from build123d import *

# Parameters (mm, degrees)
BOSS_EXTRUDE1_DEPTH     = 9.525
SKETCH3_R               = 0.508
CUT_EXTRUDE2_DEPTH      = 6.35
FILLET1_R               = 1.5875
ESQUISSE1_W             = 6.35
ESQUISSE1_H             = 6.35
BOSS_EXTRU_1_DEPTH      = 6.35
ESQUISSE2_W             = 7
ESQUISSE2_H             = 5
BOSS_EXTRU_2_DEPTH      = 15
ESQUISSE3_R             = 1.1
ENL_V_MAT_EXTRU_1_DEPTH = 58.756287679
CONG_1_R                = 2.54


with BuildPart() as part:
    # Sketch1 → Boss-Extrude1 (new body)
    with BuildSketch(Plane(origin=(0, 0, 0), x_dir=(0, 0, -1), z_dir=(1, 0, 0))):
        Polygon((0, 0), (12.7847852, 0), (12.7847852, 13.390245), (36.0778552, 13.390245), (36.0778552, 0), (48.8626404, 0), (48.8626404, 4.7625), (42.4278552, 4.7625), (42.4278552, 19.740245), (41.4309052, 19.740245), (6.3509652, 19.740245), (6.3509652, 4.7625), (0, 4.7625), align=None)
    extrude(amount=BOSS_EXTRUDE1_DEPTH)

    # Sketch3 → Cut-Extrude2 (cut)
    with BuildSketch(Plane.ZY):
        with Locations((-38.3232152, 6.68528)):
            Circle(SKETCH3_R)
        with Locations((-10.5229152, 6.6951225)):
            Circle(SKETCH3_R)
    extrude(amount=-CUT_EXTRUDE2_DEPTH, mode=Mode.SUBTRACT)

    # Fillet1
    fillet1_edges = [part.edges().sort_by_distance(p)[0] for p in [
        (4.7625, 4.7625, 0),
        (4.7625, 4.7625, -6.3509652),
        (4.7625, 19.740245, -6.3509652),
        (4.7625, 19.740245, -42.4278552),
        (4.7625, 4.7625, -42.4278552),
        (4.7625, 4.7625, -48.8626404),
    ]]
    fillet(fillet1_edges, radius=FILLET1_R)

    # Esquisse1 → Boss.-Extru.1 (add)
    with BuildSketch(Plane.XZ):
        with Locations((4.7625, -42.4702478)):
            Rectangle(ESQUISSE1_W, ESQUISSE1_H)
        with Locations((4.7625, -6.3923926)):
            Rectangle(ESQUISSE1_W, ESQUISSE1_H)
    extrude(amount=BOSS_EXTRU_1_DEPTH)

    # Esquisse2 → Boss.-Extru.2 (add)
    with BuildSketch(Plane(origin=(-5.859728485, 12.566228289, 0), x_dir=(0, 0, 1), z_dir=(0.4226182617389464, -0.9063077870374674, 0))):
        with Locations((-14.4384652, -12.4751697)):
            Rectangle(ESQUISSE2_W, ESQUISSE2_H)
    extrude(amount=-BOSS_EXTRU_2_DEPTH)

    # Esquisse3 → Enlèv. mat.-Extru.1 (cut, through all)
    with BuildSketch(Plane(origin=(9.040573976, 4.215688879, 0), x_dir=(0, 0, 1), z_dir=(-0.9063077870367755, -0.4226182617404302, 0))):
        with Locations(Location((-14.4384652, 25.865298818, 0), (0, 0, 270))):
            Circle(ESQUISSE3_R)
    extrude(amount=-ENL_V_MAT_EXTRU_1_DEPTH, mode=Mode.SUBTRACT)

    # Congé1
    # the kernel refuses this fillet: 2.54 mm, written as the material it adds along each edge
    with BuildSketch(Plane(origin=(7.318244162, 19.740245, -10.9384652), x_dir=(1, 0, 0), z_dir=(0, 0, -1))) as cong_1_piece_1:
        with BuildLine():
            CenterArc((CONG_1_R * 0.637070260809, -CONG_1_R), CONG_1_R, 90, 65)
            Line((-CONG_1_R * 0.269237526229, -CONG_1_R * 0.577381738261), (0, 0))
            Line((0, 0), (CONG_1_R * 0.637070260809, 0))
        make_face()
    extrude(amount=7)
    with BuildSketch(Plane(origin=(-4.548645433, 19.740245, -10.9384652), x_dir=(0, 0, 1), z_dir=(1, 0, 0))) as cong_1_piece_2_section:
        with BuildLine():
            CenterArc((CONG_1_R, -CONG_1_R), CONG_1_R, 90, 90)
            Line((0, -CONG_1_R), (0, 0))
            Line((0, 0), (CONG_1_R, 0))
        make_face()
    cong_1_piece_2 = extrude(amount=18.216889595, mode=Mode.PRIVATE)
    cong_1_piece_2 = split(cong_1_piece_2, bisect_by=Plane(origin=(5.198744163, 24.285527416, -10.9384652), z_dir=(-0.9063077870374674, -0.4226182617389464, 0)), keep=Keep.TOP, mode=Mode.PRIVATE)
    cong_1_piece_2 = split(cong_1_piece_2, bisect_by=Plane(origin=(0.667205228, 22.172436107, -10.9384652), z_dir=(0.9063077870374674, 0.4226182617389464, 0)), keep=Keep.TOP, mode=Mode.PRIVATE)
    add(cong_1_piece_2)
    with BuildSketch(Plane(origin=(1.801354567, 19.740245, -17.9384652), x_dir=(-1, 0, 0), z_dir=(0, 0, 1))) as cong_1_piece_3:
        with BuildLine():
            CenterArc((3.626366432, -1.766615888), CONG_1_R, 135.931485235, 69.068514765)
            Line((1.324344653, -2.840066273), (0, 0))
            Line((0, 0), (1.801354567, 0))
        make_face()
    extrude(amount=7)
    with BuildSketch(Plane(origin=(13.668244162, 19.740245, -17.9384652), x_dir=(0, 0, -1), z_dir=(-1, 0, 0))) as cong_1_piece_4_section:
        with BuildLine():
            CenterArc((CONG_1_R, -CONG_1_R), CONG_1_R, 90, 90)
            Line((0, -CONG_1_R), (0, 0))
            Line((0, 0), (CONG_1_R, 0))
        make_face()
    cong_1_piece_4 = extrude(amount=18.216889595, mode=Mode.PRIVATE)
    cong_1_piece_4 = split(cong_1_piece_4, bisect_by=Plane(origin=(8.452393501, 17.308053893, -17.9384652), z_dir=(-0.9063077870374674, -0.4226182617389464, 0)), keep=Keep.TOP, mode=Mode.PRIVATE)
    cong_1_piece_4 = split(cong_1_piece_4, bisect_by=Plane(origin=(3.920854566, 15.194962584, -17.9384652), z_dir=(0.9063077870374674, 0.4226182617389464, 0)), keep=Keep.TOP, mode=Mode.PRIVATE)
    add(cong_1_piece_4)
    with BuildSketch(Plane(origin=(7.318244162, 19.740245, -6.893069044), x_dir=(1, 0, 0), z_dir=(0, 0, -1))) as cong_1_piece_5a_section:
        with BuildLine():
            CenterArc((CONG_1_R * 0.637070260809, -CONG_1_R), CONG_1_R, 90, 65)
            Line((-CONG_1_R * 0.269237526229, -CONG_1_R * 0.577381738261), (0, 0))
            Line((0, 0), (CONG_1_R * 0.637070260809, 0))
        make_face()
    cong_1_piece_5a = extrude(amount=11.045396156, mode=Mode.PRIVATE)
    cong_1_piece_5a = split(cong_1_piece_5a, bisect_by=Plane(origin=(7.318244162, 19.740245, -10.9384652), z_dir=(0, 0, 1)), keep=Keep.TOP, mode=Mode.PRIVATE)
    with BuildSketch(Plane(origin=(-4.548645433, 19.740245, -10.9384652), x_dir=(0, 0, 1), z_dir=(1, 0, 0))) as cong_1_piece_5b_section:
        with BuildLine():
            CenterArc((CONG_1_R, -CONG_1_R), CONG_1_R, 90, 90)
            Line((0, -CONG_1_R), (0, 0))
            Line((0, 0), (CONG_1_R, 0))
        make_face()
    cong_1_piece_5b = extrude(amount=18.216889595, mode=Mode.PRIVATE)
    cong_1_piece_5b = split(cong_1_piece_5b, bisect_by=Plane(origin=(9.525, 19.740245, -10.9384652), z_dir=(-1, 0, 0)), keep=Keep.TOP, mode=Mode.PRIVATE)
    cong_1_piece_5b = split(cong_1_piece_5b, bisect_by=Plane(origin=(5.198744163, 24.285527416, -10.9384652), z_dir=(0.9063077870374674, 0.4226182617389464, 0)), keep=Keep.TOP, mode=Mode.PRIVATE)
    cong_1_piece_5 = cong_1_piece_5a & cong_1_piece_5b
    add(cong_1_piece_5)
    with BuildSketch(Plane(origin=(13.668244162, 19.740245, -17.9384652), x_dir=(0, 0, -1), z_dir=(-1, 0, 0))) as cong_1_piece_6a_section:
        with BuildLine():
            CenterArc((CONG_1_R, -CONG_1_R), CONG_1_R, 90, 90)
            Line((0, -CONG_1_R), (0, 0))
            Line((0, 0), (CONG_1_R, 0))
        make_face()
    cong_1_piece_6a = extrude(amount=18.216889595, mode=Mode.PRIVATE)
    cong_1_piece_6a = split(cong_1_piece_6a, bisect_by=Plane(origin=(9.525, 19.740245, -17.9384652), z_dir=(-1, 0, 0)), keep=Keep.TOP, mode=Mode.PRIVATE)
    cong_1_piece_6a = split(cong_1_piece_6a, bisect_by=Plane(origin=(8.452393501, 17.308053893, -17.9384652), z_dir=(0.9063077870374674, 0.4226182617389464, 0)), keep=Keep.TOP, mode=Mode.PRIVATE)
    with BuildSketch(Plane(origin=(7.318244162, 19.740245, -10.9384652), x_dir=(1, 0, 0), z_dir=(0, 0, -1))) as cong_1_piece_6b_section:
        with BuildLine():
            CenterArc((CONG_1_R * 0.637070260809, -CONG_1_R), CONG_1_R, 90, 65)
            Line((-CONG_1_R * 0.269237526229, -CONG_1_R * 0.577381738261), (0, 0))
            Line((0, 0), (CONG_1_R * 0.637070260809, 0))
        make_face()
    cong_1_piece_6b = extrude(amount=11.045396156, mode=Mode.PRIVATE)
    cong_1_piece_6b = split(cong_1_piece_6b, bisect_by=Plane(origin=(7.318244162, 19.740245, -17.9384652), z_dir=(0, 0, -1)), keep=Keep.TOP, mode=Mode.PRIVATE)
    cong_1_piece_6 = cong_1_piece_6a & cong_1_piece_6b
    add(cong_1_piece_6)
    with BuildSketch(Plane(origin=(-4.548645433, 19.740245, -10.9384652), x_dir=(0, 0, 1), z_dir=(1, 0, 0))) as cong_1_piece_7a_section:
        with BuildLine():
            CenterArc((CONG_1_R, -CONG_1_R), CONG_1_R, 90, 90)
            Line((0, -CONG_1_R), (0, 0))
            Line((0, 0), (CONG_1_R, 0))
        make_face()
    cong_1_piece_7a = extrude(amount=18.216889595, mode=Mode.PRIVATE)
    cong_1_piece_7a = split(cong_1_piece_7a, bisect_by=Plane(origin=(0, 19.740245, -10.9384652), z_dir=(1, 0, 0)), keep=Keep.TOP, mode=Mode.PRIVATE)
    cong_1_piece_7a = split(cong_1_piece_7a, bisect_by=Plane(origin=(0.667205228, 22.172436107, -10.9384652), z_dir=(-0.9063077870374674, -0.4226182617389464, 0)), keep=Keep.TOP, mode=Mode.PRIVATE)
    with BuildSketch(Plane(origin=(1.801354567, 19.740245, -17.9384652), x_dir=(-1, 0, 0), z_dir=(0, 0, 1))) as cong_1_piece_7b_section:
        with BuildLine():
            CenterArc((3.626366432, -1.766615888), CONG_1_R, 135.931485235, 69.068514765)
            Line((1.324344653, -2.840066273), (0, 0))
            Line((0, 0), (1.801354567, 0))
        make_face()
    cong_1_piece_7b = extrude(amount=14.834166034, mode=Mode.PRIVATE)
    cong_1_piece_7b = split(cong_1_piece_7b, bisect_by=Plane(origin=(1.801354567, 19.740245, -10.9384652), z_dir=(0, 0, 1)), keep=Keep.TOP, mode=Mode.PRIVATE)
    cong_1_piece_7 = cong_1_piece_7a & cong_1_piece_7b
    add(cong_1_piece_7)
    with BuildSketch(Plane(origin=(13.668244162, 19.740245, -17.9384652), x_dir=(0, 0, -1), z_dir=(-1, 0, 0))) as cong_1_piece_8a_section:
        with BuildLine():
            CenterArc((CONG_1_R, -CONG_1_R), CONG_1_R, 90, 90)
            Line((0, -CONG_1_R), (0, 0))
            Line((0, 0), (CONG_1_R, 0))
        make_face()
    cong_1_piece_8a = extrude(amount=18.216889595, mode=Mode.PRIVATE)
    cong_1_piece_8a = split(cong_1_piece_8a, bisect_by=Plane(origin=(0, 19.740245, -17.9384652), z_dir=(1, 0, 0)), keep=Keep.TOP, mode=Mode.PRIVATE)
    cong_1_piece_8a = split(cong_1_piece_8a, bisect_by=Plane(origin=(3.920854566, 15.194962584, -17.9384652), z_dir=(-0.9063077870374674, -0.4226182617389464, 0)), keep=Keep.TOP, mode=Mode.PRIVATE)
    with BuildSketch(Plane(origin=(1.801354567, 19.740245, -25.772631234), x_dir=(-1, 0, 0), z_dir=(0, 0, 1))) as cong_1_piece_8b_section:
        with BuildLine():
            CenterArc((3.626366432, -1.766615888), CONG_1_R, 135.931485235, 69.068514765)
            Line((1.324344653, -2.840066273), (0, 0))
            Line((0, 0), (1.801354567, 0))
        make_face()
    cong_1_piece_8b = extrude(amount=14.834166034, mode=Mode.PRIVATE)
    cong_1_piece_8b = split(cong_1_piece_8b, bisect_by=Plane(origin=(1.801354567, 19.740245, -17.9384652), z_dir=(0, 0, -1)), keep=Keep.TOP, mode=Mode.PRIVATE)
    cong_1_piece_8 = cong_1_piece_8a & cong_1_piece_8b
    add(cong_1_piece_8)
    # the kernel refuses this fillet: 2.54 mm, written as the material it takes off along each edge
    with BuildSketch(Plane(origin=(7.128164948, 35.173251244, -17.9384652), x_dir=(0, 0, 1), z_dir=(-0.9063077870374675, -0.42261826173894645, 0)), Plane(origin=(-8.913482883, 27.692908011, -10.9384652), x_dir=(0, 0, -1), z_dir=(0.9063077870374675, 0.42261826173894645, 0))) as cong_1_2_piece_1:
        with BuildLine():
            CenterArc((CONG_1_R, -CONG_1_R), CONG_1_R, 90, 90)
            Line((0, -CONG_1_R), (0, 0))
            Line((0, 0), (CONG_1_R, 0))
        make_face()
    extrude(amount=17.7, mode=Mode.SUBTRACT)


solid = part.part
Build history of the part. All positions in model axes, mm. A direction names the side the tool comes from. Give positions to 0.01 mm unless a question says otherwise; leave off trailing zeros. Loops run counter-clockwise (first coordinate to the right, second up) from the corner with the lowest first, then second, coordinate; pieces in that order, holes last. Notation, with made-up numbers: (63, 77.5) - (88, 77.5) arc R20 ccw to (88, 110.5) - close; hole circle Ø10 at (71.25, 71.5). An arc over 180 degrees is marked (long way). Write item = value, one per line. Start each with the question number.
1) Band-saw the part on A-A on y = 12. Give the cut face in (x, z) (3 decimals).
2) Drop flat-ended pins along their axis: pin 1 Ø6.5 at (x, y) = (2.5, 28) entering from -Z; pin 2 Ø2.5 at (x, z) = (2.5, -45) entering from +Y; pin 3 Ø6 at (x, z) = (1.5, -34) entering from -Y; pin 4 Ø3 at (y, z) = (17, -5.5) entering from +X (3 decimals). Give the stop position or say it passes through.
3) Band-saw the part on B-B on x = 4. Count the separate pieces of the cut face and the enclosed holes in it, plus the area to 3 significant figures.
4) Tool access for faces 1 (the cylindrical face through (3.13, 6.38, -38.73)), 2 (the flat face through (5, -3, -45.645)), 3 (the flat face through (5, 4.762, -46)), 4 (the flat face through (7.938, -3, -43)): list every direction of +Z, -Z, +X, -X, +Y, -Y with a clear straight run to the whole face (end or side of a thin tool).
5) Probe probe 1 along Z at (x, y) = (7.5, -3); probe 2 along Z at (x, y) = (2, 9); probe 3 along X at (y, z) = (13, -8.5) (3 decimals). List the from-to ranges inside material, lowest first. Write a range as from..to.
6) Pull direction Z, two halves, no side cores. Call faces 5 (the flat face through (2, 25, -10.938)), 6 (the cylindrical face through (0.24, 28.92, -15.51)), 7 (the cylindrical face through (4.829, 4.285, -48.41)): +Z half, -Z half, draft (parallel to the pull), parting line (faces both ways), or undercut.
Final values:
q1.outline = (0, -42.428) - (9.525, -42.428) - (9.525, -36.078) - (0, -36.078) - close; (0, -12.785) - (9.525, -12.785) - (9.525, -6.351) - (0, -6.351) - close
q2.pin_1 = -17.94
q2.pin_2 = 4.78
q2.pin_3 = 0
q2.pin_4 = 9.525
q3.separate_pieces = 1
q3.enclosed_holes = 2
q3.area = 592 mm²
q4.face_1 = -X
q4.face_2 = -Z, +X, -X, -Y
q4.face_3 = -Z, +X, -X, +Y
q4.face_4 = +Z, -Z, +X, -Y
q5.probe_1 = -45.65..-39.3, -9.57..-3.22
q5.probe_2 = -42.43..-36.08, -12.78..-6.35
q5.probe_3 = 0..9.525
q6.face_5 = +Z half
q6.face_6 = undercut
q6.face_7 = -Z half
